Source: CAD feature listing. Evaluate the final solid. Frame: model axes, mm. Coordinates: 2 decimals unless noted, no trailing zeros. Order: outer loops, then holes, each group sorted by start corner. A loop starts at its lowest first (then second) coordinate and runs counter-clockwise, first axis right, second up.
Autodesk Inventor part; units mm, degrees
ref_plane "YZ Plane" through (0, 0, 0) normal (1, 0, 0) x (0, 1, 0)
ref_plane "XZ Plane" through (0, 0, 0) normal (0, 1, 0) x (-1, 0, 0)
ref_plane "XY Plane" through (0, 0, 0) normal (0, 0, 1) x (1, 0, 0)
sketch "Sketch1" plane through (0, 0, 0) normal (0, 0, 1) x (1, 0, 0)
  circle A0 centre (0, 0) radius 46.5667
  circle A1 centre (0, 0) radius 19.05
  dimension "d0" = 93.1333
  dimension "d1" = 38.1
extrude "Extrusion1" add sketch "Sketch1" along normal blind 6.35
sketch "Sketch2" plane through (0, 0, 6.35) normal (0, 0, 1) x (1, 0, 0)
  line L0 (21.1667, 36.6617) -> (42.3333, 0) construction
  line L1 (42.3333, 0) -> (21.1667, -36.6617) construction
  line L2 (21.1667, -36.6617) -> (-21.1667, -36.6617) construction
  line L3 (-21.1667, -36.6617) -> (-42.3333, 0) construction
  line L4 (-42.3333, 0) -> (-21.1667, 36.6617) construction
  line L5 (-21.1667, 36.6617) -> (21.1667, 36.6617) construction
  line L6 (-21.1667, 36.6617) -> (-23.2833, 40.3279) construction
  circle A0 centre (0, 0) radius 46.5667 construction
  dimension "d4" = 4.2333
hole "Hole1" at (-21.1667, 36.6617, 6.35) at (-42.3333, 0, 6.35) at (-21.1667, -36.6617, 6.35) at (42.3333, 0, 6.35) at (21.1667, -36.6617, 6.35) at (21.1667, 36.6617, 6.35) direction (0, 0, -1) diameter 6 end through all
properties part number "Stator Front"
1. Section query D-D on z = 1.5. Return loops of the section in (x, y), plus the area to 3 significant figures.
Findings:
outline: circle Ø93.13 at (0, 0); hole circle Ø6 at (-42.33, 0); hole circle Ø6 at (-21.17, -36.66); hole circle Ø6 at (-21.17, 36.66); hole circle Ø38.1 at (0, 0); hole circle Ø6 at (21.17, -36.66); hole circle Ø6 at (21.17, 36.66); hole circle Ø6 at (42.33, 0)
area: 5,500 mm2
2. Pin query (flat end, axial travel): P1, Ø6, axis at x = 2, y = 21.5, coming from the -Z side; P2, Ø1.5, axis at x = -23, z = 5.5, coming from the -Y side. Return the tip coordinate at first contact, or that it passes through.
Findings:
P1: stops at z = 0
P2: stops at y = -40.91
3. Section query C-C on y = -11. Return loops of the section in (x, z).
Findings:
outline: (-45.25, 0) - (-15.55, 0) - (-15.55, 6.35) - (-45.25, 6.35) - close; (15.55, 0) - (45.25, 0) - (45.25, 6.35) - (15.55, 6.35) - close
4. Section query A-A on x = 0. Return loops of the section in (y, z), plus the area to 3 significant figures.
Findings:
outline: (-46.57, 0) - (-19.05, 0) - (-19.05, 6.35) - (-46.57, 6.35) - close; (19.05, 0) - (46.57, 0) - (46.57, 6.35) - (19.05, 6.35) - close
area: 349 mm2
5. Draft query along Y for faces 1 (the face through (20, 1, 6.35)), 2 (the face through (-20.018, -39.433, 3.131)), 3 (the face through (-10.09, 45.46, 3.13)). Return one class per face: released by +Y, released by -Y, zero draft, split by the parting line, or undercut.
Findings:
face 1: zero draft
face 2: undercut
face 3: split by the parting line
6. Ray query, line 1 (Y direction, x = 0, z = 2.25); line 2 (X direction, y = -2.5, z = 2.5); line 3 (Y direction, x = 22.5, z = 3). Return the intervals inside material, ascending.
Findings:
line 1: y = -46.57 to -19.05, 19.05 to 46.57
line 2: x = -46.5 to -43.99, -40.67 to -18.89, 18.89 to 40.67, 43.99 to 46.5
line 3: y = -40.77 to -39.35, -33.97 to 33.97, 39.35 to 40.77
7. Section query B-B on y = 0. Return loops of the section in (x, z).
Findings:
outline: (-46.57, 0) - (-45.33, 0) - (-45.33, 6.35) - (-46.57, 6.35) - close; (-39.33, 0) - (-19.05, 0) - (-19.05, 6.35) - (-39.33, 6.35) - close; (19.05, 0) - (39.33, 0) - (39.33, 6.35) - (19.05, 6.35) - close; (45.33, 0) - (46.57, 0) - (46.57, 6.35) - (45.33, 6.35) - close
